from build123d import *

# Parameters (mm, degrees)
F0_R     = 1.5875
F0_R_2   = 3.175
F1_DEPTH = 13
F2_W     = 6.35
F2_H     = 19.05
F3_DEPTH = 37.5
F4_R     = 6.35
F5_R     = 2.54
F6_SIZE  = 3.175


# Not quite as in the source:
# - a feature names something its author has since deleted; it is built from what else it names


with BuildPart() as f1:
    # F0 (on Right) → F1 (new body)
    with BuildSketch(Plane.YZ):
        Polygon((0, 0), (0, -12.7), (92.075, -12.7), (92.075, 0), (92.075, 12.7), (0, 12.7), align=None)
        with Locations((6.35, 0)):
            Circle(F0_R, mode=Mode.SUBTRACT)
        with Locations((19.05, 0)):
            Circle(F0_R, mode=Mode.SUBTRACT)
        with Locations((41.275, 0)):
            Circle(F0_R_2, mode=Mode.SUBTRACT)
        with Locations((82.55, 0)):
            Circle(F0_R, mode=Mode.SUBTRACT)
    extrude(amount=-F1_DEPTH)

    # F2 (on Top) → F3 (cut, symmetric)
    with BuildSketch(Plane.XY):
        with BuildLine():
            Line((0, 30.2764773719), (0, 52.2735226281))
            ThreePointArc((0, 52.2735226281), (-6.35, 41.275), (0, 30.2764773719))
        make_face()
        with Locations((-3.175, 82.55)):
            Rectangle(F2_W, F2_H)
    extrude(amount=F3_DEPTH, both=True, mode=Mode.SUBTRACT)

    # F4
    f4_edges = [f1.edges().sort_by_distance(p)[0] for p in [
        (-6.5, 0, -12.7),
        (-6.5, 0, 12.7),
        (-9.675, 92.075, -12.7),
        (-9.675, 92.075, 12.7),
    ]]
    fillet(f4_edges, radius=F4_R)

    # F5
    f5_edges = [f1.edges().sort_by_distance(p)[0] for p in [
        (-13, 90.215128, -10.840128),
        (-13, 92.075, 0),
        (0, 0, 0),
        (0, 62.649261, 12.7),
        (0, 62.649261, -12.7),
        (-13, 0, 0),
        (0, 1.859872, -10.840128),
        (0, 1.859872, 10.840128),
        (0, 18.313239, -12.7),
        (0, 18.313239, 12.7),
        (-13, 1.859872, -10.840128),
        (-13, 1.859872, 10.840128),
        (-13, 46.0375, -12.7),
        (-13, 90.215128, 10.840128),
        (-13, 46.0375, 12.7),
    ]]
    fillet(f5_edges, radius=F5_R)

    # F6
    f6_edges = [f1.edges().sort_by_distance(p)[0] for p in [
        (-13, 38.1, 0),
    ]]
    chamfer(f6_edges, length=F6_SIZE)


solid = f1.part
Geometry check sheet. Reference: the model listing, model coordinates, mm. A direction names the side the tool comes from. Round coordinates to 2 decimals unless told otherwise and drop trailing zeros. Order: outer loops, then holes, each group sorted by start corner. A loop starts at its lowest first (then second) coordinate and runs counter-clockwise, first axis right, second up. Notation, with made-up numbers: M 5,-4 L 48,-4 A17 ccw 48,11 Z; hole C -14.5,11.25 d10. An arc over 180 degrees is marked long. Answer in a Markdown table with one row per item.
(1) Draft check along Y on faces 3 (the face through (-9.98, 44.35, -1.28)), 4 (the face through (0, 63, 0)), 5 (the face through (-12.276, 0.764, -0.089)). Enter one of: released by +Y, released by -Y, zero draft, split by the parting line, or undercut.
Responses:
| item | result |
|---|---|
| face 3 | undercut |
| face 4 | zero draft |
| face 5 | released by -Y |
(2) Sectioned sample at A-A, the plane x = -4.25. State how many separate pieces and enclosed holes the cut face has, and give its area (3 significant figures).
Responses:
| item | result |
|---|---|
| separate pieces | 2 |
| enclosed holes | 2 |
| area | 1,470 mm² |
(3) Go/stop test with flat-tipped pins: P1, Ø1.9, axis at x = -1.5, z = 0.5, coming from the +Y side (3 decimals); P2, Ø2.5, axis at y = 82.55, z = 0, coming from the +X side; P3, Ø9.5, axis at y = 86.5, z = 0.5, coming from the +X side; P4, Ø1, axis at x = -7, z = -8.5, coming from the -Y side. Record where each tip stops, or that it passes through.
Responses:
| item | result |
|---|---|
| P1 | stops at y = 73.025 |
| P2 | passes through |
| P3 | stops at x = -6.35 |
| P4 | stops at y = 0.22 |
(4) Scan lines: probe 1 along Z at (x, y) = (-8, 19.05); probe 2 along Y at (x, z) = (-4.25, 1) (3 decimals); probe 3 along Z at (x, y) = (-12, 37). Record each from-to range of solid material in increasing order. Write a range as from..to.
Responses:
| item | result |
|---|---|
| probe 1 | z = -12.7..-1.59, 1.59..12.7 |
| probe 2 | y = 0..5.117, 7.583..17.817, 20.283..34.28, 48.27..73.025 |
| probe 3 | z = -12.18..-3.22, 3.22..12.18 |
(5) Tool access check on faces 1 (the face through (-0.724, 61.526, 11.936)), 2 (the face through (-3, 73.025, 0)). Record the directions out of +Z, -Z, +X, -X, +Y, -Y that give a thin tool (end or side, any length) a straight path to the whole face; none if there is none.
Responses:
| item | result |
|---|---|
| face 1 | +Z, +X, +Y, -Y |
| face 2 | +Z, -Z, +X, +Y |
(6) Sectioned sample at C-C, the plane y = 82.55. Record the cut outline in (x, z).
Responses:
| item | result |
|---|---|
| outline | M -13,-10.16 A2.54 ccw -10.46,-12.7 L -6.35,-12.7 L -6.35,-1.59 L -13,-1.59 Z; M -13,1.59 L -6.35,1.59 L -6.35,12.7 L -10.46,12.7 A2.54 ccw -13,10.16 Z |
